from build123d import *

# Parameters (mm, degrees)
F1_DEPTH = 11.45
F2_R     = 13.25
F3_DEPTH = 22.901
F6_SIZE  = 2.7


with BuildPart() as f1:
    # F0 (on Top) → F1 (new body, symmetric)
    with BuildSketch(Plane.XY):
        Polygon((12.606495, -22.84928), (26.091305, -0.507095), (13.484809, 22.342185), (-12.606495, 22.84928), (-26.091305, 0.507095), (-13.484809, -22.342185), align=None)
    extrude(amount=F1_DEPTH, both=True)

    # F2 (on face) → F3 (cut, through all)
    with BuildSketch(Plane.XY.offset(11.45)):
        Circle(F2_R)
    extrude(amount=-F3_DEPTH, mode=Mode.SUBTRACT)

    # F4 (on Front) → F5 (revolve, cut)
    with BuildSketch(Plane.XZ):
        Polygon((34.293845, 11.45), (21.591305, 11.45), (26.091305, 8.75), (26.091305, -8.75), (21.591305, -11.45), (34.293845, -11.45), align=None)
    revolve(axis=Axis((0, 0, 11.45), (0, 0, 1)), mode=Mode.SUBTRACT)

    # F6
    f6_edges = [f1.edges().sort_by_distance(p)[0] for p in [
        (-13.25, 0, 11.45),
        (-13.25, 0, -11.45),
    ]]
    chamfer(f6_edges, length=F6_SIZE)


solid = f1.part
Read the model definition and answer for the solid it produces. Units are mm, in the model's axes. Round coordinates to 2 decimals unless told otherwise and drop trailing zeros. Write each loop counter-clockwise with the first axis right and the second up, starting at its lowest first coordinate (ties: lowest second). Pieces come first, ordered by that corner, then holes. Notation, with made-up numbers: M 60.25,79 L 91.25,79 A15 ccw 91.25,94 Z; hole C 33,-34 d8. An arc over 180 degrees is marked long. Use a Markdown table: item, result.
1) Flat-ended cylindrical pins translate along their axes: pin 1 (8 mm diameter, centred on x = -21, y = -12.5, fed in from -Z); pin 2 (1.5 mm diameter, centred on x = 6.5, z = 7, fed in from +Y); pin 3 (1.5 mm diameter, centred on x = 15.5, z = -8, fed in from +Y); pin 4 (2 mm diameter, centred on y = -4.5, z = 0, fed in from -X). Find the tip coordinate at first contact, or state that the pin passes through.
Answers follow:
| item | result |
|---|---|
| pin 1 | stops at z = -11.45 |
| pin 2 | stops at y = 22.49 |
| pin 3 | stops at y = 20.05 |
| pin 4 | stops at x = -23.88 |
2) The part is cut by section B-B (x = 0). Write down the section's boundary in (y, z).
Answers follow:
| item | result |
|---|---|
| outline | M -22.6,-10.84 L -21.59,-11.45 L -15.95,-11.45 L -13.25,-8.75 L -13.25,8.75 L -15.95,11.45 L -21.59,11.45 L -22.6,10.84 Z; M 13.25,-8.75 L 15.95,-11.45 L 21.59,-11.45 L 22.6,-10.84 L 22.6,10.84 L 21.59,11.45 L 15.95,11.45 L 13.25,8.75 Z |
3) For a pull along X with two mould halves and no side action, classify faces 1 (the conical face through (-2.9, -13.06, 8.88)), 2 (the flat face through (-2, -16, 11.45)), 3 (the cylindrical face through (7.123, 11.172, 0.123)), 4 (the flat face through (-19.255, 11.834, 0.152)) as pulls with the +X half, pulls with the -X half, needs draft (parallel to the pull), parting line crosses it, or undercut.
Answers follow:
| item | result |
|---|---|
| face 1 | undercut |
| face 2 | needs draft |
| face 3 | undercut |
| face 4 | pulls with the -X half |
4) Straight lines are drawn through the part: line 1 along Y through (x, z) = (0, -3); line 2 along Y through (x, z) = (-9, 1.5); line 3 along X through (y, z) = (0.5, -7). For each, find the intervals that lie inside material, in ascending order. Write a range as [from, to].
Answers follow:
| item | result |
|---|---|
| line 1 | y = [-22.6, -13.25], [13.25, 22.6] |
| line 2 | y = [-22.43, -9.72], [9.72, 22.78] |
| line 3 | x = [-26.09, -13.24], [13.24, 25.54] |
